from build123d import *

# Parameters (mm, degrees)
SKETCH012_W  = 39
SKETCH012_H  = 5
PAD012_DEPTH = 14
PAD013_DEPTH = 20
SKETCH014_R  = 4.5
PAD014_DEPTH = 35
CHAMFER_SIZE = 2
SKETCH015_R  = 2.5
POCKET_DEPTH = 10


with BuildPart() as part:
    # Sketch012 → Pad012 (new body)
    with BuildSketch(Plane.XY.offset(0.5)):
        with Locations((0, 52.5)):
            Rectangle(SKETCH012_W, SKETCH012_H)
    extrude(amount=PAD012_DEPTH)

    # Sketch013 → Pad013 (join)
    with BuildSketch(Plane.YZ.offset(-10)):
        Polygon((40, 14), (35, 9), (35, 6), (40, 1), (50, 1), (50, 14), align=None)
    extrude(amount=PAD013_DEPTH)

    # Sketch014 → Pad014 (join)
    with BuildSketch(Plane.XZ.offset(-50)):
        with Locations((-12.5, 7.5)):
            Circle(SKETCH014_R)
        with Locations((12.5, 7.5)):
            Circle(SKETCH014_R)
    extrude(amount=PAD014_DEPTH)

    # Chamfer
    chamfer_edges = [part.edges().sort_by_distance(p)[0] for p in [
        (8, 15, 7.5),
        (-17, 15, 7.5),
        (19.5, 50, 7.5),
        (19.5, 55, 7.5),
        (19.5, 52.5, 0.5),
        (19.5, 52.5, 14.5),
        (-19.5, 55, 7.5),
        (-19.5, 50, 7.5),
        (-19.5, 52.5, 0.5),
        (-19.5, 52.5, 14.5),
    ]]
    chamfer(chamfer_edges, length=CHAMFER_SIZE)

    # Sketch015 → Pocket (cut)
    with BuildSketch(Plane.XZ.offset(-55)):
        with Locations((-12.5, 7.5)):
            Circle(SKETCH015_R)
        with Locations((0, 7.5)):
            Circle(SKETCH015_R)
        with Locations((12.5, 7.5)):
            Circle(SKETCH015_R)
    extrude(amount=POCKET_DEPTH, mode=Mode.SUBTRACT)


with BuildPart() as part_1:
    # Body004 placement: moved
    add(part.part.moved(Location((0, 5, -30))))


solid = part_1.part
Could you check a few things on this model? Use its own coordinates, in mm. A direction names the side the tool comes from. Round coordinates to 2 decimals unless told otherwise and drop trailing zeros. Order: outer loops, then holes, each group sorted by start corner. A loop starts at its lowest first (then second) coordinate and runs counter-clockwise, first axis right, second up. Notation, with made-up numbers: M 88.5,82 L 133.5,82 A15 ccw 133.5,93 Z; hole C -6,40 d2. An arc over 180 degrees is marked long. One line per item, written item: value.
(1) I'm going to push flat-ended pins straight in: P1, Ø0.8, axis at y = 51.5, z = -17.5, coming from the +X side; P2, Ø1.5, axis at x = -11.5, y = 44, coming from the -Z side; P3, Ø1.4, axis at y = 49, z = -27, coming from the -X side; P4, Ø11, axis at x = 4.5, y = 51, coming from the +Z side. Where does each tip first touch, or does it pass through?
Ans:
P1: stops at x = 10
P2: stops at z = -26.99
P3: stops at x = -14.91
P4: stops at z = -15.5
(2) If we mould it in two halves opening along Z, with no side actions, what happens to faces 4 (the flat face through (0, 50, -22)), 5 (the cylindrical face through (10.66, 55.07, -20.81)), 6 (the flat face through (-18.5, 56, -22.6)), 7 (the flat face through (0, 58, -29.5))? For each: released by +Z, released by -Z, zero draft, split by the parting line, or undercut.
Ans:
face 4: undercut
face 5: undercut
face 6: zero draft
face 7: released by -Z
(3) Imagine slicing it at B-B (x = 0). Write out the boundary of the cut face in (y, z).
Ans:
outline: M 40,-24 L 45,-29 L 55,-29 L 55,-29.5 L 60,-29.5 L 60,-25 L 50,-25 L 50,-20 L 60,-20 L 60,-15.5 L 55,-15.5 L 55,-16 L 45,-16 L 40,-21 Z
(4) Which directions (+Z, -Z, +X, -X, +Y, -Y) give clear straight access to the entire face, cutting with the end or side of a thin tool? Please do faces 1 (the flat face through (-0.1, 55, -15.8)), 2 (the flat face through (0, 42, -26)), 3 (the flat face through (10, 49, -17)).
Ans:
face 1: -Y
face 2: -Z, -Y
face 3: +Z, -Y
(5) Imagine slicing it at A-A (y = 44.5). Write out the boundary of the cut face in (x, z), and give its area (3 significant figures).
Ans:
outline: M -10,-28.5 L 10,-28.5 L 10,-26.24 A4.5 ccw long 10,-18.76 L 10,-16.5 L -10,-16.5 L -10,-18.76 A4.5 ccw long -10,-26.24 Z
area: 346 mm^2
(6) Imagine slicing it at D-D (y = 25). Write out the boundary of the cut face in (x, z), and give its area (3 significant figures).
Ans:
outline: C -12.5,-22.5 d9; C 12.5,-22.5 d9
area: 127 mm^2
(7) I need wall thicknesses on line 1 along Z through (x, y) = (12.5, 56); line 2 along Z through (x, y) = (-12.5, 54.25); line 3 along Z through (x, y) = (10, 31.5). Which ranges of each line are inside material? Lowest first, please. Write a range as from..to.
Ans:
line 1: z = -29.5..-25, -20..-15.5
line 2: z = -27..-25, -20..-18
line 3: z = -26.24..-18.76
